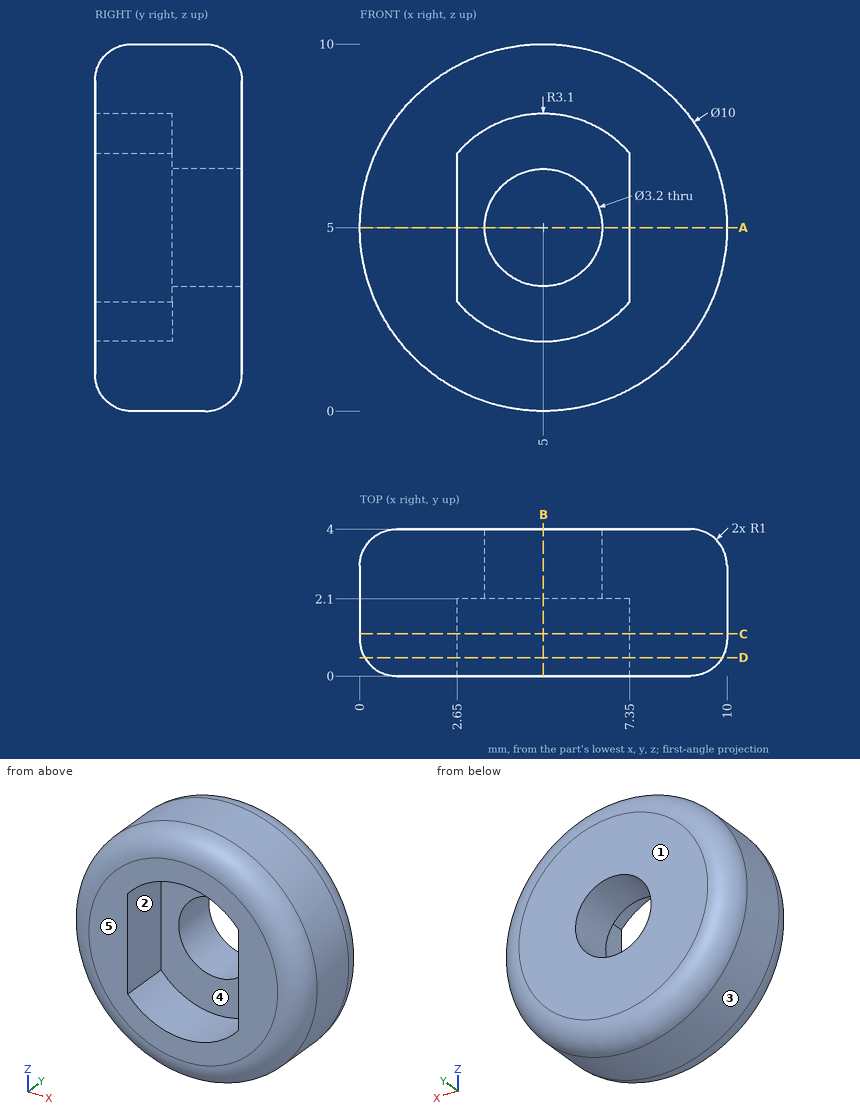
Can you work these out from the drawing? Everything is in mm from the part's minimum corner. A direction names the side the tool comes from. Coordinates: 2 decimals unless noted, no trailing zeros. Loops run counter-clockwise (first coordinate to the right, second up) from the corner with the lowest first, then second, coordinate; pieces in that order, holes last. Notation, with made-up numbers: (-27.5, 32) - (27.5, 32) arc R28 cw to (27.5, 62) - close; hole circle Ø8 at (7, -11.75). An arc over 180 degrees is marked (long way). Put each result on its own line as item: value. Start each with the question number.
Item 1: Suppose I cut it at C-C (y = 1.15). Please give me the cut outline in (x, z).
Item 2: If we mould it in two halves opening along X, with no side actions, what happens to the marked faces 1, 2 and 3? For each: +X half, -X half, draft (parallel to the pull), parting line (faces both ways), or undercut.
Item 3: Which directions (+Z, -Z, +X, -X, +Y, -Y) give clear straight access to the entire face, cutting with the end or side of a thin tool? Please do the marked faces 4 and 5.
Item 4: Suppose I cut it at B-B (x = 5). Please give me the cut outline in (y, z).
Item 5: For pin 1 (1 mm diameter, centred on y = 1, z = 6, fed in from -X); pin 2 (2 mm diameter, centred on y = 1, z = 3.5, fed in from +X); pin 3 (2 mm diameter, centred on y = 3.5, z = 8, fed in from -X), each with a flat end and sliding along its axis, tell me the tip position at first contact or that it passes through.
Item 6: If I drill on line 1 along X through (y, z) = (2.75, 5); line 2 along Y through (x, z) = (5.5, 7); line 3 along X through (y, z) = (1.75, 2.5), over which ranges is the centre line in solid material (lowest first)?
Item 7: Suppose I cut it at D-D (y = 0.5). Please give me the cut outline in (x, z), and give its area (3 significant figures).
Item 8: Suppose I cut it at A-A (z = 5). Please give me the cut outline in (x, y).
Here are the results:
1. outline: circle Ø10 at (5, 5); hole (2.65, 2.98) arc R3.1 ccw to (7.35, 2.98) - (7.35, 7.02) arc R3.1 ccw to (2.65, 7.02) - close
2. face 1: draft
2. face 2: undercut
2. face 3: parting line
3. face 4: -Y
3. face 5: +Z, -Z, +X, -X, -Y
4. outline: (0, 1) arc R1 ccw to (1, 0) - (3, 0) arc R1 ccw to (4, 1) - (4, 3.4) - (2.1, 3.4) - (2.1, 1.9) - (0, 1.9) - close; (0, 8.1) - (2.1, 8.1) - (2.1, 6.6) - (4, 6.6) - (4, 9) arc R1 ccw to (3, 10) - (1, 10) arc R1 ccw to (0, 9) - close
5. pin 1: x = 0.03
5. pin 2: x = 9.97
5. pin 3: x = 0.46
6. line 1: 0 to 3.4, 6.6 to 10
6. line 2: 2.1 to 4
6. line 3: 0.67 to 3.17, 6.83 to 9.33
7. outline: circle Ø9.73 at (5, 5); hole (2.65, 2.98) arc R3.1 ccw to (7.35, 2.98) - (7.35, 7.02) arc R3.1 ccw to (2.65, 7.02) - close
7. area: 48.3 mm²
8. outline: (0, 1) arc R1 ccw to (1, 0) - (2.65, 0) - (2.65, 2.1) - (3.4, 2.1) - (3.4, 4) - (1, 4) arc R1 ccw to (0, 3) - close; (6.6, 2.1) - (7.35, 2.1) - (7.35, 0) - (9, 0) arc R1 ccw to (10, 1) - (10, 3) arc R1 ccw to (9, 4) - (6.6, 4) - close
